from build123d import *

# Parameters (mm, degrees)
SKETCH1_R           = 19.05
BOSS_EXTRUDE2_DEPTH = 3.175
SKETCH2_R           = 14.2875
BOSS_EXTRUDE3_DEPTH = 12.7
SKETCH5_R           = 12.7
BOSS_EXTRUDE4_DEPTH = 6.35
SKETCH6_W           = 44.45
SKETCH6_H           = 53.975
BOSS_EXTRUDE5_DEPTH = 6.35
SKETCH7_W           = 44.45
SKETCH7_H           = 6.35
BOSS_EXTRUDE6_DEPTH = 34.925
SKETCH8_W           = 38.1
SKETCH8_H           = 25.4
BOSS_EXTRUDE7_DEPTH = 12.7
SKETCH9_W           = 28.575
SKETCH9_H           = 4.343134019
BOSS_EXTRUDE9_DEPTH = 25.4


with BuildPart() as part:
    # Sketch1 → Boss-Extrude2 (new body)
    with BuildSketch(Plane.XY):
        Circle(SKETCH1_R)
    extrude(amount=BOSS_EXTRUDE2_DEPTH)

    # Sketch2 → Boss-Extrude3 (add)
    with BuildSketch(Plane.XY.offset(3.175)):
        Circle(SKETCH2_R)
    extrude(amount=BOSS_EXTRUDE3_DEPTH)

    # Sketch5 → Boss-Extrude4 (add)
    with BuildSketch(Plane.XY.offset(15.875)):
        Circle(SKETCH5_R)
    extrude(amount=BOSS_EXTRUDE4_DEPTH)

    # Sketch6 → Boss-Extrude5 (add)
    with BuildSketch(Plane.XY.offset(22.225)):
        with Locations((0, -6.486273282)):
            Rectangle(SKETCH6_W, SKETCH6_H)
    extrude(amount=BOSS_EXTRUDE5_DEPTH)

    # Sketch7 → Boss-Extrude6 (add)
    with BuildSketch(Plane.XY.offset(28.575)):
        with Locations((0, -30.298773282)):
            Rectangle(SKETCH7_W, SKETCH7_H)
    extrude(amount=BOSS_EXTRUDE6_DEPTH)

    # Sketch8 → Boss-Extrude7 (add)
    with BuildSketch(Plane.XY.offset(28.575)):
        with Locations((0, 0.181226718)):
            Rectangle(SKETCH8_W, SKETCH8_H)
    extrude(amount=BOSS_EXTRUDE7_DEPTH)

    # Sketch9 → Boss-Extrude9 (add)
    with BuildSketch(Plane.XY.offset(41.275)):
        with Locations((0, -10.347206273)):
            Rectangle(SKETCH9_W, SKETCH9_H)
    extrude(amount=BOSS_EXTRUDE9_DEPTH)


solid = part.part
Can you work these out from the model? Positions are in its coordinate system, mm. A direction names the side the tool comes from. Round coordinates to 2 decimals unless told otherwise and drop trailing zeros. Loops run counter-clockwise (first coordinate to the right, second up) from the corner with the lowest first, then second, coordinate; pieces in that order, holes last. Notation, with made-up numbers: (33, 87.25) - (59, 87.25) arc R25 cw to (59, 114.25) - close; hole circle Ø6 at (-21.5, -37.75). An arc over 180 degrees is marked (long way). Write item = value, one per line. Start each with the question number.
(1) If we section it at C-C (y = 17): Please give me the cut outline in (x, z) (3 decimals).
(2) If we mould it in two halves opening along Z, with no side actions, what happens to faces 5 (the face through (-13, -1, 15.875)), 6 (the face through (-15.12, -11.59, 1.57)), 7 (the face through (0, 0, 0))? For each: released by +Z, released by -Z, zero draft, split by the parting line, or undercut.
(3) If we section it at A-A (z = 31.5): Please give me the cut outline in (x, y) (3 decimals), and give its area (3 significant figures).
(4) If we section it at D-D (y = -5): Please give me the cut outline in (x, z) (3 decimals).
(5) For faces 1 (the face through (0, -30, 63.5)), 2 (the face through (0, 12.881, 35)), 3 (the face through (14.288, -10, 54)), 4 (the face through (2.7, 14.2, 3.175)), which set-ups out of +Z, -Z, +X, -X, +Y, -Y let a thin tool reach every point of the face, with its end or its side?
(6) If I drill on probe 1 along Y at (x, z) = (-1.5, 53); probe 2 along Z at (x, y) = (-10, -26) (3 decimals); probe 3 along Z at (x, y) = (2.5, -28) (3 decimals), over which ranges is the centre line in solid material (lowest first)? Write a range as [from, to].
(7) For P1, Ø5, axis at y = -10, z = 51.5, coming from the -X side; P2, Ø23, axis at x = 2, y = 4.5, coming from the +Z side (3 decimals); P3, Ø10, axis at y = -8.5, z = 48.5, coming from the +X side, each with a flat end and sliding along its axis, tell me the tip position at first contact or that it passes through.
Ans:
q1.outline = (-22.225, 22.225) - (22.225, 22.225) - (22.225, 28.575) - (-22.225, 28.575) - close; (-8.597, 0) - (8.597, 0) - (8.597, 3.175) - (-8.597, 3.175) - close
q2.face_5 = undercut
q2.face_6 = zero draft
q2.face_7 = released by -Z
q3.outline = (-22.225, -33.474) - (22.225, -33.474) - (22.225, -27.124) - (-22.225, -27.124) - close; (-19.05, -12.519) - (19.05, -12.519) - (19.05, 12.881) - (-19.05, 12.881) - close
q3.area = 1,250 mm²
q4.outline = (-22.225, 22.225) - (-11.674, 22.225) - (-11.674, 15.875) - (-13.384, 15.875) - (-13.384, 3.175) - (-18.382, 3.175) - (-18.382, 0) - (18.382, 0) - (18.382, 3.175) - (13.384, 3.175) - (13.384, 15.875) - (11.674, 15.875) - (11.674, 22.225) - (22.225, 22.225) - (22.225, 28.575) - (19.05, 28.575) - (19.05, 41.275) - (-19.05, 41.275) - (-19.05, 28.575) - (-22.225, 28.575) - close
q5.face_1 = +Z, +X, -X, -Y
q5.face_2 = +Z, +X, -X, +Y
q5.face_3 = +Z, +X, +Y
q5.face_4 = none
q6.probe_1 = [-33.47, -27.12], [-12.52, -8.18]
q6.probe_2 = [22.225, 28.575]
q6.probe_3 = [22.225, 63.5]
q7.P1 = -14.29
q7.P2 = 41.275
q7.P3 = 14.29
